Check sheet for the modelled part. Datum: model origin and axes. Units: mm. Round coordinates to 2 decimals unless told otherwise and drop trailing zeros. Write each loop counter-clockwise with the first axis right and the second up, starting at its lowest first coordinate (ties: lowest second). Pieces come first, ordered by that corner, then holes. Notation, with made-up numbers: (-27.5, 55) - (13.5, 55) arc R12 ccw to (13.5, 66) - close; hole circle Ø11 at (14.5, -2.75). An arc over 180 degrees is marked (long way). Answer as a JSON object with one key per item and string values. Group by question number.
Item 1: Release check for a two-part mould opening along Y. For faces 1 (the flat face through (-9, 175, 1)), 2 (the flat face through (0, 0, 1)), 3 (the flat face through (-21.38, 94.84, 1.48)) record: pulls with the +Y half, pulls with the -Y half, needs draft (parallel to the pull), parting line crosses it, or undercut.
Item 2: Sectioned sample at D-D on x = 25.5. Record the boundary of the cut face in (y, z).
Item 3: Gauge pin test, flat ends, axial feed: P1, Ø1, axis at x = -17, z = 2, coming from the +Y side; P2, Ø1.5, axis at y = 45, z = 2, coming from the +X side. Record the tip position at first contact, or that the pin passes through.
Item 4: Sectioned sample at C-C on y = 21. Record the boundary of the cut face in (x, z), plus the area to 3 significant figures.
Item 5: Sectioned sample at A-A on y = 146. Record the boundary of the cut face in (x, z), plus the area to 3 significant figures.
Item 6: Thickness scan on line 1 (X direction, y = 81.5, z = 2.1); line 2 (X direction, y = 126, z = 1.85); line 3 (X direction, y = 56.5, z = 0.25). Record the ranges inside material, lowest first.
Item 7: Sectioned sample at B-B on x = 7.5. Record the boundary of the cut face in (y, z), plus the area to 3 significant figures.
```python
from build123d import *

# Parameters (mm, degrees)
F1_DEPTH = 3
F4_DEPTH = 4.85
F3_R     = 0.775
F5_DEPTH = 1.8
F6_R     = 1.5
F7_R     = 0.775


with BuildPart() as f1:
    # F0 (on Top) → F1 (new body)
    with BuildSketch(Plane.XY):
        with BuildLine():
            Line((-14.4016106971, 0), (0, 0))
            Line((0, 0), (14.4016106971, 0))
            ThreePointArc((14.4016106971, 0), (25.530513069, 4.9427870661), (29.3250428137, 16.5136624004))
            Line((29.3250428137, 16.5136624004), (13.25, 175))
            Line((13.25, 175), (4.25, 175))
            Line((4.25, 175), (2.0357756631, 83.826056716))
            ThreePointArc((2.0357756631, 83.826056716), (11.9564350998, 70.9784033555), (0, 60))
            ThreePointArc((0, 60), (-11.9564350998, 70.9784033555), (-2.0357756631, 83.826056716))
            Line((-2.0357756631, 83.826056716), (-4.25, 175))
            Line((-4.25, 175), (-13.25, 175))
            Line((-13.25, 175), (-29.3250428137, 16.5136624004))
            ThreePointArc((-29.3250428137, 16.5136624004), (-25.530513069, 4.9427870661), (-14.4016106971, 0))
        make_face()
    extrude(amount=F1_DEPTH)

    # F3 (on offset) → F4 (join)
    with BuildSketch(Plane.YZ.offset(13.25)):
        with BuildLine():
            ThreePointArc((171.0013200045, 0), (172.0619801762, 0.4393398282), (172.5013200045, 1.5))
            ThreePointArc((172.5013200045, 1.5), (169.9406598327, 2.5606601718), (171.0013200045, 0))
        make_face()
    extrude(amount=F4_DEPTH)

    # F3 (on offset) → F5 (join)
    with BuildSketch(Plane.YZ.offset(13.25)):
        with Locations((167.0013200045, 1.5)):
            Circle(F3_R)
    extrude(amount=F5_DEPTH)

    # F6
    f6_edges = [f1.edges().sort_by_distance(p)[0] for p in [
        (18.1, 171.00132, 3),
    ]]
    fillet(f6_edges, radius=F6_R)

    # F7
    f7_edges = [f1.edges().sort_by_distance(p)[0] for p in [
        (15.05, 166.22632, 1.5),
    ]]
    fillet(f7_edges, radius=F7_R)

    # F8: F1 across plane


with BuildPart() as f1_1:
    add(f1.part)
    add(f1.part.mirror(Plane.YZ))


solid = f1_1.part
```
Completed:
{
 "1": {"face 1": "pulls with the +Y half", "face 2": "pulls with the -Y half", "face 3": "undercut"},
 "2": {"outline": "(4.91, 0) - (54.23, 0) - (54.23, 3) - (4.91, 3) - close"},
 "3": {"P1": "y = 172.49", "P2": "x = 26.51"},
 "4": {"outline": "(-28.87, 0) - (28.87, 0) - (28.87, 3) - (-28.87, 3) - close", "area": "173 mm²"},
 "5": {"outline": "(-16.19, 0) - (-3.55, 0) - (-3.55, 3) - (-16.19, 3) - close; (3.55, 0) - (16.19, 0) - (16.19, 3) - (3.55, 3) - close", "area": "75.9 mm²"},
 "6": {"line 1": "-22.73 to -7.33, 7.33 to 22.73", "line 2": "-18.22 to -3.06, 3.06 to 18.22", "line 3": "-25.27 to 25.27"},
 "7": {"outline": "(0, 0) - (62.63, 0) - (62.63, 3) - (0, 3) - close; (81.37, 0) - (175, 0) - (175, 3) - (81.37, 3) - close", "area": "469 mm²"}
}
